Geometry check sheet. Reference: the model listing, model coordinates, mm. Face numbers are marked on the shaded views. A direction names the side the tool comes from. Coordinates: 2 decimals unless noted, no trailing zeros. Loops run counter-clockwise (first coordinate to the right, second up) from the corner with the lowest first, then second, coordinate; pieces in that order, holes last.
Autodesk Inventor part; units mm, degrees
ref_plane "YZ Plane" through (0, 0, 0) normal (1, 0, 0) x (0, 1, 0)
ref_plane "XZ Plane" through (0, 0, 0) normal (0, 1, 0) x (-1, 0, 0)
ref_plane "XY Plane" through (0, 0, 0) normal (0, 0, 1) x (1, 0, 0)
sketch "Sketch1" plane through (0, 0, 0) normal (0, 1, 0) x (-1, 0, 0)
  line L0 (0, 0) -> (-114.3, 0)
  line L1 (-114.3, 0) -> (-114.3, 152.4)
  line L2 (-114.3, 152.4) -> (0, 152.4)
  line L3 (0, 152.4) -> (0, 0)
  line L4 (-57.15, 34.925) -> (-69.85, 34.925)
  line L5 (-69.85, 34.925) -> (-69.85, 47.625)
  line L6 (-69.85, 47.625) -> (-57.15, 47.625)
  line L7 (-57.15, 47.625) -> (-57.15, 34.925)
  line L8 (-57.15, 104.775) -> (-69.85, 104.775)
  line L9 (-69.85, 104.775) -> (-69.85, 117.475)
  line L10 (-69.85, 117.475) -> (-57.15, 117.475)
  line L11 (-57.15, 117.475) -> (-57.15, 104.775)
  dimension "d0" = 152.4
  dimension "d1" = 114.3
  dimension "d2" = 12.7
  dimension "d3" = 12.7
  dimension "d4" = 12.7
  dimension "d5" = 12.7
  dimension "d6" = 34.925
  dimension "d7" = 34.925
  dimension "d8" = 44.45
  dimension "d9" = 44.45
extrude "Extrusion1" add sketch "Sketch1" along normal blind 10.16
sketch "Sketch2" plane through (0, 0, 0) normal (-1, 0, 0) x (0, 0, 1)
  line L0 (0, 10.16) -> (152.4, 10.16)
  line L1 (53.975, 10.16) -> (98.425, 10.16)
  line L2 (98.425, 10.16) -> (98.425, 22.86)
  line L3 (98.425, 22.86) -> (93.345, 22.86)
  line L4 (93.345, 22.86) -> (93.345, 19.05)
  line L5 (93.345, 19.05) -> (86.614, 10.16)
  line L6 (86.614, 10.16) -> (76.2, 10.16)
  line L7 (65.786, 10.16) -> (59.055, 19.05)
  line L8 (59.055, 19.05) -> (59.055, 22.86)
  line L9 (59.055, 22.86) -> (53.975, 22.86)
  line L10 (53.975, 22.86) -> (53.975, 10.16)
  line L11 (0, 0) -> (0, 10.16)
  dimension "d12" = 0
  dimension "d13" = 20.828
  dimension "d14" = 44.45
  dimension "d15" = 3.81
  dimension "d16" = 3.81
  dimension "d17" = 12.7
  dimension "d18" = 12.7
  dimension "d19" = 5.08
  dimension "d20" = 5.08
  dimension "d21" = 11.811
  dimension "d24" = 53.975
extrude "Extrusion2" add sketch "Sketch2" against normal blind 63.5
sketch "Sketch4" plane through (0, 10.16, 0) normal (0, 1, 0) x (1, 0, 0)
  circle A0 centre (20.32, -47.625) radius 3.81
  circle A1 centre (44.45, -47.625) radius 3.81
  circle A2 centre (20.32, -104.775) radius 3.81
  circle A3 centre (44.45, -104.775) radius 3.81
  line L0 (0, -53.975) -> (63.5, -53.975)
  line L1 (63.5, -98.425) -> (0, -98.425)
  line L2 (0, -98.425) -> (0, -152.4)
  line L3 (0, 0) -> (0, -53.975)
  dimension "d28" = 7.62
  dimension "d29" = 7.62
  dimension "d30" = 7.62
  dimension "d31" = 7.62
  dimension "d32" = 6.35
  dimension "d33" = 6.35
  dimension "d34" = 6.35
  dimension "d35" = 6.35
  dimension "d36" = 20.32
  dimension "d37" = 44.45
  dimension "d38" = 20.32
  dimension "d39" = 44.45
extrude "Extrusion4" cut sketch "Sketch4" against normal blind 10.16
sketch "Sketch5" plane through (0, 0, 152.4) normal (0, 0, 1) x (1, 0, 0)
  line L0 (0, 0) -> (114.3, 0)
  line L1 (0, 10.16) -> (114.3, 10.16)
  line L2 (114.3, 10.16) -> (114.3, 0)
  line L3 (114.3, 0) -> (0, 0)
  line L4 (0, 0) -> (0, 10.16)
extrude "Extrusion5" add sketch "Sketch5" along normal blind 25.4
sketch "Sketch6" plane through (114.3, 0, 0) normal (0, 0, -1) x (-1, 0, 0)
  line L0 (0, 10.16) -> (114.3, 10.16)
  line L1 (114.3, 0) -> (0, 0)
  line L2 (0, 10.16) -> (114.3, 10.16)
  line L3 (114.3, 10.16) -> (114.3, 0)
  line L4 (114.3, 0) -> (0, 0)
  line L5 (0, 0) -> (0, 10.16)
extrude "Extrusion6" add sketch "Sketch6" along normal blind 25.4
sketch "Sketch7" plane through (0, 10.16, 0) normal (0, 1, 0) x (1, 0, 0)
  line L0 (114.3, 25.4) -> (114.3, -177.8)
  line L1 (114.3, -98.425) -> (101.6, -98.425)
  line L2 (101.6, -98.425) -> (101.6, -53.975)
  line L3 (101.6, -53.975) -> (114.3, -53.975)
  line L4 (114.3, -53.975) -> (114.3, -98.425)
  line L5 (0, -98.425) -> (63.5, -98.425)
  line L6 (0, -53.975) -> (63.5, -53.975)
  point P0 (0, 0)
  dimension "d46" = 0
  dimension "d47" = 0
  dimension "d48" = 12.7
extrude "Extrusion7" add sketch "Sketch7" along normal blind 12.7
sketch "Sketch8" plane through (0, 10.16, 0) normal (0, 1, 0) x (1, 0, 0)
  line L0 (114.3, -177.8) -> (0, -177.8)
  line L1 (80.01, -177.8) -> (92.71, -177.8)
  line L2 (92.71, -177.8) -> (92.71, -76.2)
  line L3 (92.71, -76.2) -> (80.01, -76.2)
  line L4 (80.01, -76.2) -> (80.01, -177.8)
  line L5 (101.6, -98.425) -> (101.6, -53.975)
  point P0 (0, 0)
  dimension "d51" = 8.89
  dimension "d52" = 12.7
  dimension "d53" = 101.6
extrude "Extrusion8" cut sketch "Sketch8" against normal blind 3.175
sketch "Sketch9" plane through (0, 0, 0) normal (0, -1, 0) x (1, 0, 0)
  line L0 (0, 177.8) -> (0, -25.4)
  line L1 (114.3, 177.8) -> (92.71, 177.8)
  line L2 (0, -25.4) -> (114.3, -25.4)
  line L3 (114.3, -25.4) -> (114.3, 177.8)
  line L4 (114.3, 177.8) -> (0, 177.8)
  line L5 (0, 177.8) -> (0, -25.4)
  point P0 (0, 0)
extrude "Extrusion9" cut sketch "Sketch9" against normal blind 3.81
sketch "Sketch10" plane through (0, 10.16, 0) normal (0, 1, 0) x (1, 0, 0)
  circle A0 centre (71.12, -144.145) radius 3.81
  circle A1 centre (101.6, -144.145) radius 3.81
  line L0 (0, -93.345) -> (63.5, -93.345)
  line L1 (92.71, -76.2) -> (92.71, -177.8)
  line L2 (80.01, -177.8) -> (80.01, -76.2)
  point P0 (0, 0)
  dimension "d58" = 50.8
  dimension "d59" = 50.8
  dimension "d60" = 7.62
  dimension "d61" = 7.62
  dimension "d68" = 8.89
  dimension "d69" = 8.89
extrude "Extrusion10" cut sketch "Sketch10" against normal blind 25.4
sketch "Sketch13" plane through (0, 22.86, 59.055) normal (0, 1, 0) x (1, 0, 0)
  line L0 (0, 0) -> (63.5, 0)
  line L1 (0, -34.29) -> (63.5, -34.29)
  line L2 (0, 0) -> (4.953, 0)
  line L3 (4.953, 0) -> (4.953, -34.29)
  line L4 (4.953, -34.29) -> (0, -34.29)
  line L5 (0, -34.29) -> (0, 0)
  point P0 (0, 59.055)
  dimension "d70" = 4.953
extrude "Extrusion13" add sketch "Sketch13" against normal blind 12.7
sketch "Sketch14" plane through (4.953, 22.86, 93.345) normal (1, 0, 0) x (0, 0, -1)
  line L0 (11.176, -2.032) -> (23.114, -2.032)
  line L1 (23.114, -2.032) -> (23.114, -7.62)
  line L2 (23.114, -7.62) -> (11.176, -7.62)
  line L3 (11.176, -7.62) -> (11.176, -2.032)
  line L4 (27.559, -12.7) -> (6.731, -12.7)
  point P0 (93.345, -22.86)
  dimension "d73" = 5.08
  dimension "d74" = 5.588
  dimension "d75" = 4.445
  dimension "d76" = 4.445
extrude "Extrusion14" cut sketch "Sketch14" against normal blind 12.7
sketch "Sketch15" plane through (0, 10.16, 0) normal (0, 1, 0) x (1, 0, 0)
  line L0 (101.6, -98.425) -> (92.71, -98.425)
  line L1 (92.71, -98.425) -> (92.71, -53.975)
  line L2 (92.71, -53.975) -> (101.6, -53.975)
  line L3 (101.6, -53.975) -> (101.6, -98.425)
  line L4 (101.6, -53.975) -> (114.3, -53.975)
  line L5 (92.71, -76.2) -> (92.71, -177.8)
  point P0 (0, 0)
  point P1 (92.71, -176.403)
  dimension "d79" = 0
  dimension "d80" = 0
extrude "Extrusion15" add sketch "Sketch15" along normal blind 9.9568
chamfer "Chamfer1" distance 8.89 angle 45 1 edges at (92.71, 20.1168, 76.2)
sketch "Sketch19" plane through (0, 10.16, 0) normal (0, 1, 0) x (1, 0, 0)
  line L0 (114.3, 25.4) -> (88.9, 25.4)
  line L1 (114.3, 25.4) -> (0, 25.4)
  line L2 (88.9, 17.78) -> (97.79, 17.78)
  line L3 (97.79, 17.78) -> (97.79, 0)
  line L4 (97.79, 0) -> (105.41, 0)
  line L5 (105.41, 0) -> (105.41, 17.78)
  line L6 (105.41, 17.78) -> (114.3, 17.78)
  line L7 (114.3, -177.8) -> (114.3, 25.4)
  line L8 (114.3, 17.78) -> (114.3, 25.4)
  line L9 (88.9, 17.78) -> (88.9, 25.4)
  line L10 (63.5, 25.4) -> (63.5, 17.78)
  line L11 (63.5, 17.78) -> (54.61, 17.78)
  line L12 (54.61, 17.78) -> (54.61, 0)
  line L13 (54.61, 0) -> (46.99, 0)
  line L14 (46.99, 0) -> (46.99, 17.78)
  line L15 (46.99, 17.78) -> (38.1, 17.78)
  line L16 (38.1, 17.78) -> (38.1, 25.4)
  line L17 (63.5, 25.4) -> (38.1, 25.4)
  point P0 (0, 0)
  dimension "d118" = 25.4
  dimension "d119" = 25.4
  dimension "d120" = 25.4
  dimension "d121" = 7.62
  dimension "d122" = 7.62
  dimension "d123" = 8.89
  dimension "d124" = 7.62
  dimension "d125" = 17.78
  dimension "d126" = 17.78
  dimension "d127" = 7.62
  dimension "d128" = 8.89
extrude "Extrusion18" add sketch "Sketch19" along normal blind 25.4
chamfer "Chamfer4" distance 17.78 distance2 25.4 1 edges at (50.8, 35.56, 0) measured on face at (52.07, 35.56, -22.86)
chamfer "Chamfer5" distance 17.78 distance2 25.4 1 edges at (101.6, 35.56, 0) measured on face at (100.33, 35.56, -22.86)
sketch "Sketch20" plane through (54.61, 10.16, -17.78) normal (0, 0, 1) x (1, 0, 0)
  line L0 (-16.51, 25.4) -> (-7.62, 25.4)
  line L1 (-16.51, 0) -> (-16.51, 25.4)
  line L2 (0, 25.4) -> (8.89, 25.4)
  line L3 (8.89, 0) -> (8.89, 25.4)
  line L4 (34.29, 0) -> (34.29, 25.4)
  line L5 (34.29, 25.4) -> (43.18, 25.4)
  line L6 (50.8, 25.4) -> (59.69, 25.4)
  line L7 (59.69, 0) -> (59.69, 25.4)
  point P0 (-54.61, -10.16)
  point P1 (-11.43, 20.32)
  point P2 (3.81, 20.32)
  point P3 (39.37, 20.32)
  point P4 (54.61, 20.32)
  dimension "d137" = 5.08
  dimension "d138" = 5.08
  dimension "d139" = 5.08
  dimension "d140" = 5.08
  dimension "d141" = 5.08
  dimension "d142" = 5.08
  dimension "d143" = 5.08
  dimension "d144" = 5.08
hole "Hole1" at (43.18, 30.48, -17.78) at (58.42, 30.48, -17.78) at (93.98, 30.48, -17.78) at (109.22, 30.48, -17.78) direction (0, 0, -1) diameter 5.08 end through all
properties part number "Elevator Slide Top"
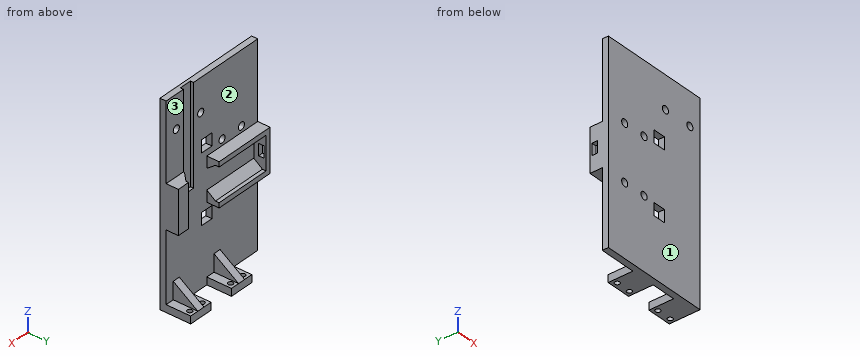
(1) Sectioned sample at C-C on x = 20.32. Record the cut outline in (y, z) (3 decimals).
Findings:
outline: (3.81, -25.4) - (10.16, -25.4) - (10.16, 43.815) - (3.81, 43.815) - close; (3.81, 51.435) - (10.16, 51.435) - (10.16, 53.975) - (22.86, 53.975) - (22.86, 59.055) - (19.05, 59.055) - (10.16, 65.786) - (10.16, 86.614) - (19.05, 93.345) - (22.86, 93.345) - (22.86, 98.425) - (10.16, 98.425) - (10.16, 100.965) - (3.81, 100.965) - close; (3.81, 108.585) - (10.16, 108.585) - (10.16, 177.8) - (3.81, 177.8) - close
(2) Sectioned sample at B-B on y = 30.48. State how many separate pieces and enclosed holes the cut face has, and give its area (3 significant figures).
Findings:
separate pieces: 6
enclosed holes: 0
area: 286 mm2
(3) Access from +Z, -Z, +X, -X, +Y, -Y to the whole of each face (thin tool, end or side, straight path). Record for the marked faces 1, 2 and 3.
Findings:
face 1: +Z, -Z, +X, -X, -Y
face 2: +Y
face 3: +Z, +X, -X, +Y
(4) Sectioned sample at A-A on x = 109.22. Record the cut outline in (y, z) (3 decimals), and give its area (3 significant figures).
Findings:
outline: (3.81, -25.4) - (27.94, -25.4) - (27.94, -17.78) - (10.16, -17.78) - (10.16, 53.975) - (22.86, 53.975) - (22.86, 98.425) - (10.16, 98.425) - (10.16, 177.8) - (3.81, 177.8) - close; (33.02, -25.4) - (35.56, -25.4) - (35.56, -17.78) - (33.02, -17.78) - close
area: 2,010 mm2
(5) Gauge pin test, flat ends, axial feed: pin 1 Ø1 at (x, z) = (57, 26.5) entering from +Y; pin 2 Ø5 at (x, z) = (35.5, 97.5) entering from +Y; pin 3 Ø14 at (x, y) = (24.5, 18) entering from -Z (3 decimals). Record the tip position at first contact, or that the pin passes through.
Findings:
pin 1: stops at y = 10.16
pin 2: stops at y = 22.86
pin 3: stops at z = 53.975
(6) Scan lines: L1, parallel to Z at x = 44.45, y = 7.25 (3 decimals); L2, parallel to X at y = 30.48, z = -19.75; L3, parallel to X at y = 20.5, z = 62. Record each from-to range of solid material in increasing order.
Findings:
L1: z = -25.4 to 43.815, 51.435 to 100.965, 108.585 to 177.8
L2: x = 38.1 to 40.64, 45.72 to 55.88, 60.96 to 63.5, 88.9 to 91.44, 96.52 to 106.68, 111.76 to 114.3
L3: x = 0 to 4.95, 101.6 to 114.3
